from build123d import *

# Parameters (mm, degrees)
BOX012_W                    = 13
BOX012_H                    = 65
BOX012_DEPTH                = 1
CYLINDER004_R               = 4
CYLINDER004_DEPTH           = 10
CYLINDER002_R               = 1.45
CYLINDER002_DEPTH           = 10
CYLINDER001_R               = 2.35
CYLINDER001_DEPTH           = 15
CYLINDER001_PLACEMENT_ANGLE = 45
CYLINDER_R                  = 1.45
CYLINDER_DEPTH              = 10
BOX004_W                    = 8
BOX004_H                    = 20
BOX004_DEPTH                = 15
BOX002_W                    = 13
BOX002_H                    = 25.5
BOX002_DEPTH                = 9
BOX003_W                    = 13
BOX003_H                    = 25
BOX003_DEPTH                = 50
BOX003_PLACEMENT_ANGLE      = 45
BOX_W                       = 13
BOX_H                       = 20
BOX_DEPTH                   = 20
BOX001_W                    = 13
BOX001_H                    = 65
BOX001_DEPTH                = 35
CHAMFER_SIZE                = 1
FILLET_R                    = 4


with BuildPart() as cube008:
    # Box012 → Box012 (new body)
    with BuildSketch(Plane(origin=(0, -20, 0), x_dir=(1, 0, 0), z_dir=(0, 0, 1))):
        with Locations((6.5, 32.5)):
            Rectangle(BOX012_W, BOX012_H)
    extrude(amount=BOX012_DEPTH)


with BuildPart() as cylinder004:
    # Cylinder004 → Cylinder004 (new body)
    with BuildSketch(Plane(origin=(0, 37.5, 6), x_dir=(0, 0, -1), z_dir=(1, 0, 0))):
        Circle(CYLINDER004_R)
    extrude(amount=CYLINDER004_DEPTH)


with BuildPart() as cylinder002:
    # Cylinder002 → Cylinder002 (new body)
    with BuildSketch(Plane(origin=(8, -11, 25.5), x_dir=(1, 0, 0), z_dir=(0, -1, 0))):
        Circle(CYLINDER002_R)
    extrude(amount=CYLINDER002_DEPTH)


with BuildPart() as cylinder001:
    # Cylinder001 → Cylinder001 (new body)
    with BuildSketch(Plane.XY):
        Circle(CYLINDER001_R)
    extrude(amount=CYLINDER001_DEPTH)


with BuildPart() as cylinder001_1:
    # Cylinder001 placement: moved
    add(cylinder001.part.moved(Location((6.5, -8.899495, 4.343146))).rotate(Axis((6.5, -8.899495, 4.343146), (-1, 0, 0)), CYLINDER001_PLACEMENT_ANGLE))


with BuildPart() as fusion_holes:
    # Cylinder → Cylinder (new body)
    with BuildSketch(Plane(origin=(8, 30, 18), x_dir=(1, 0, 0), z_dir=(0, 0, 1))):
        Circle(CYLINDER_R)
    extrude(amount=CYLINDER_DEPTH)

    # Fusion001: union Cylinder002, Cylinder001
    add(cylinder002.part)
    add(cylinder001_1.part)


with BuildPart() as cube003:
    # Box004 → Box004 (new body)
    with BuildSketch(Plane(origin=(0, 25, 0), x_dir=(1, 0, 0), z_dir=(0, 0, 1))):
        with Locations((4, 10)):
            Rectangle(BOX004_W, BOX004_H)
    extrude(amount=BOX004_DEPTH)


with BuildPart() as cube002:
    # Box002 → Box002 (new body)
    with BuildSketch(Plane(origin=(0, 19.5, 26), x_dir=(1, 0, 0), z_dir=(0, 0, 1))):
        with Locations((6.5, 12.75)):
            Rectangle(BOX002_W, BOX002_H)
    extrude(amount=BOX002_DEPTH)


with BuildPart() as cube_45deg:
    # Box003 → Box003 (new body)
    with BuildSketch(Plane.XY):
        with Locations((6.5, 12.5)):
            Rectangle(BOX003_W, BOX003_H)
    extrude(amount=BOX003_DEPTH)


with BuildPart() as cube_45deg_1:
    # Box003 placement: moved
    add(cube_45deg.part.moved(Location((0, -18.485281, -18.384776))).rotate(Axis((0, -18.485281, -18.384776), (1, 0, 0)), BOX003_PLACEMENT_ANGLE))


with BuildPart() as fusion:
    # Box → Box (new body)
    with BuildSketch(Plane.XY):
        with Locations((6.5, 10)):
            Rectangle(BOX_W, BOX_H)
    extrude(amount=BOX_DEPTH)

    # Fusion: union Cube002, cube_45deg
    add(cube002.part)
    add(cube_45deg_1.part)


with BuildPart() as body:
    # Box001 → Box001 (new body)
    with BuildSketch(Plane(origin=(0, -20, 0), x_dir=(1, 0, 0), z_dir=(0, 0, 1))):
        with Locations((6.5, 32.5)):
            Rectangle(BOX001_W, BOX001_H)
    extrude(amount=BOX001_DEPTH)

    # Cut: cut Fusion
    add(fusion.part, mode=Mode.SUBTRACT)

    # Cut001: cut Cube003
    add(cube003.part, mode=Mode.SUBTRACT)

    # Cut002: cut fusion holes
    add(fusion_holes.part, mode=Mode.SUBTRACT)

    # Fusion002: union Cylinder004
    add(cylinder004.part)

    # Cut008: cut Cube008
    add(cube008.part, mode=Mode.SUBTRACT)

    # Chamfer
    chamfer_edges = [body.edges().sort_by_distance(p)[0] for p in [
        (6.5, 45, 26),
        (6.5, 19.5, 35),
        (6.5, -20, 35),
        (6.5, 0, 1),
        (6.5, 20, 1),
    ]]
    chamfer(chamfer_edges, length=CHAMFER_SIZE)

    # Fillet
    fillet_edges = [body.edges().sort_by_distance(p)[0] for p in [
        (10.5, 45, 1),
        (4, 25, 15),
    ]]
    fillet(fillet_edges, radius=FILLET_R)


solid = body.part
Source: CAD feature listing. Evaluate the final solid. Frame: model axes, mm. A direction names the side the tool comes from. Give positions to 0.01 mm unless a question says otherwise; leave off trailing zeros. Loops run counter-clockwise (first coordinate to the right, second up) from the corner with the lowest first, then second, coordinate; pieces in that order, holes last. Notation, with made-up numbers: (-7.5, 64) -> (42.5, 64) arc R9 ccw to (42.5, 69) -> close; hole circle Ø5 at (80, 57.5). An arc over 180 degrees is marked (long way). Use a Markdown table: item, result. Add a question column.
1) Section query C-C, the plane x = 10.75. Return the cut outline in (y, z).
2) First-contact query: pin 1 (2.5 mm diameter, centred on x = 5, y = 34.5, fed in from -Z); pin 2 (15.5 mm diameter, centred on y = 30.5, z = 6.5, fed in from -X); pin 3 (1.5 mm diameter, centred on x = 2.5, z = 30, fed in from +Y); pin 4 (6 mm diameter, centred on x = 3, y = 36, fed in from +Z). Flat tips, straight axial feed; report the tip coordinate or a pass-through.
3) Section query A-A, the plane y = 37.5. Return the cut outline in (x, z).
4) Pull-direction query (Z, two-part tool) for faces 1 (the face through (9, 29, 1)), 2 (the face through (8, -11, 26)), 3 (the face through (6, 0, 9)); classes: +Z half, -Z half, draft (parallel to the pull), parting line (faces both ways), or undercut.
5) Line query: line 1 along X through (y, z) = (30, 23); line 2 along Y through (x, z) = (8, 22.75); line 3 along Z through (x, y) = (1.75, 21). Output: solid intervals per line, ascending. Write a range as [from, to].
6) Reachability of faces 4 (the face through (6.85, -15.44, 24.62)), 5 (the face through (6, 20, 11)), 6 (the face through (4, 25, 6)), 7 (the face through (8, 34.9, 9.5)) from +Z, -Z, +X, -X, +Y, -Y: full face, straight path, thin tool, end or side. Return the list, or none.
7) Section query B-B, the plane x = 7.25. Count the separate pieces of the cut face and the enclosed holes in it, then the cut area to 3 significant figures.
8) Section query D-D, the plane y = 30. Return the cut outline in (x, z), then the cut area to 3 significant figures.
Numbers:
| question | item | result |
|---|---|---|
| 1 | outline | (-20, 18.49) -> (-2.51, 1) -> (-1, 1) -> (0, 2) -> (0, 20) -> (20, 20) -> (20, 2) -> (21, 1) -> (41, 1) arc R4 ccw to (45, 5) -> (45, 25) -> (44, 26) -> (19.5, 26) -> (19.5, 34) -> (18.5, 35) -> (-19, 35) -> (-20, 34) -> close |
| 2 | pin 1 | stops at z = 2.4 |
| 2 | pin 2 | stops at x = 0 |
| 2 | pin 3 | stops at y = 19.5 |
| 2 | pin 4 | stops at z = 26 |
| 3 | outline | (0, 2) -> (8, 2) -> (8, 1) -> (13, 1) -> (13, 26) -> (0, 26) -> (0, 15) -> (8, 15) -> (8, 10) -> (0, 10) -> close |
| 4 | face 1 | -Z half |
| 4 | face 2 | undercut |
| 4 | face 3 | draft |
| 5 | line 1 | x = [0, 6.55], [9.45, 13] |
| 5 | line 2 | y = [-20, 28.55], [31.45, 45] |
| 5 | line 3 | z = [1, 26] |
| 6 | face 4 | -Y |
| 6 | face 5 | -Z, +X, -X |
| 6 | face 6 | -Z, -X |
| 6 | face 7 | -X |
| 7 | separate pieces | 3 |
| 7 | enclosed holes | 0 |
| 7 | area | 1,130 mm2 |
| 8 | outline | (0, 15) -> (8, 15) -> (8, 1) -> (13, 1) -> (13, 26) -> (9.45, 26) -> (9.45, 18) -> (6.55, 18) -> (6.55, 26) -> (0, 26) -> close |
| 8 | area | 190 mm2 |
